Geometry: see drawing. Coordinates: mm, zero at the bounding-box minimum. Round coordinates to 2 decimals unless told otherwise and drop trailing zeros. Order: outer loops, then holes, each group sorted by start corner. A loop starts at its lowest first (then second) coordinate and runs counter-clockwise, first axis right, second up.
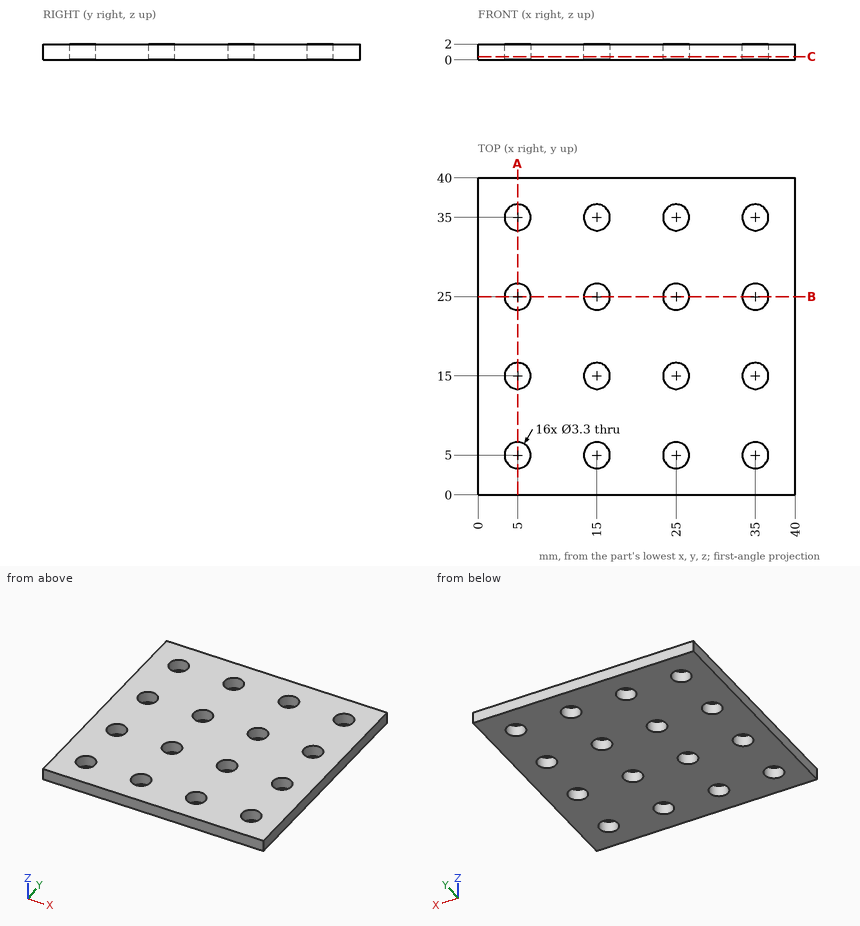
1. Line query: line 1 along Y through (x, z) = (5, 1.55); line 2 along Y through (x, z) = (6.5, 1.3); line 3 along X through (y, z) = (35.5, 0.45). Output: solid intervals per line, ascending.
2. Section C-C on z = 0.4. State how many separate pieces and enclosed holes the cut face has, plus the area to 3 significant figures.
3. Section A-A on x = 5. Return loops of the section in (y, z), plus the area to 3 significant figures.
4. First-contact query: pin 1 (2 mm diameter, centred on x = 25, y = 5, fed in from +Z). Flat tip, straight axial feed; report the tip coordinate or a pass-through.
Result:
1. line 1: y = 0 to 3.35, 6.65 to 13.35, 16.65 to 23.35, 26.65 to 33.35, 36.65 to 40
1. line 2: y = 0 to 4.31, 5.69 to 14.31, 15.69 to 24.31, 25.69 to 34.31, 35.69 to 40
1. line 3: x = 0 to 3.43, 6.57 to 13.43, 16.57 to 23.43, 26.57 to 33.43, 36.57 to 40
2. separate pieces: 1
2. enclosed holes: 16
2. area: 1,460 mm2
3. outline: (0, 0) - (3.35, 0) - (3.35, 2) - (0, 2) - close; (6.65, 0) - (13.35, 0) - (13.35, 2) - (6.65, 2) - close; (16.65, 0) - (23.35, 0) - (23.35, 2) - (16.65, 2) - close; (26.65, 0) - (33.35, 0) - (33.35, 2) - (26.65, 2) - close; (36.65, 0) - (40, 0) - (40, 2) - (36.65, 2) - close
3. area: 53.6 mm2
4. pin 1: passes through
